from build123d import *

# Parameters (mm, degrees)
F0_R            = 31.75
F1_DEPTH        = 6.35
F2_R            = 4.7625
F3_DEPTH        = 6.351
F3_COPIES_COUNT = 6
F4_R            = 3.175
F5_R            = 3.175
F6_DEPTH        = 6.3510001
F6_COPIES_COUNT = 6
F7_R            = 9.4615
F7_R_2          = 7.9375
F8_DEPTH        = 9.7028
F8_COPIES_COUNT = 6


# Not quite as in the source:
# - a pattern or mirror of a feature is missing from the dataset's text; its kind, count and spacing are read off the source's solid


with BuildPart() as f1:
    # F0 (on Front) → F1 (new body)
    with BuildSketch(Plane.XZ):
        Circle(F0_R)
    extrude(amount=F1_DEPTH)

    # F2 (on face) → F3 (cut, through all)
    with BuildSketch(Plane.XZ.offset(6.35)):
        with Locations((-15.875, 27.4963065702)):
            Circle(F2_R)
    f3 = extrude(amount=-F3_DEPTH, mode=Mode.SUBTRACT)

    # F3_copies: F3 ×6 about axis
    f3_copies_axis = Axis((0, 0, 0), (0, 1, 0))
    for i in range(1, F3_COPIES_COUNT):
        add(f3.rotate(f3_copies_axis, i * 360 / F3_COPIES_COUNT), mode=Mode.SUBTRACT)

    # F4
    f4_edges = [f1.edges().sort_by_distance(p)[0] for p in [
        (-19.809236, -3.175, 24.81243),
        (-11.583577, -3.175, 29.561516),
        (-31.392813, -3.175, 4.749087),
        (11.583577, -3.175, 29.561516),
        (19.809236, -3.175, 24.81243),
        (31.392813, -3.175, 4.749087),
        (31.392813, -3.175, -4.749087),
        (19.809236, -3.175, -24.81243),
        (11.583577, -3.175, -29.561516),
        (-11.583577, -3.175, -29.561516),
        (-19.809236, -3.175, -24.81243),
        (-31.392813, -3.175, -4.749087),
    ]]
    fillet(f4_edges, radius=F4_R)

    # F5 (on face) → F6 (cut, through all)
    with BuildSketch(Plane.XZ.offset(6.35)):
        with Locations((0, 20.6375)):
            Circle(F5_R)
    f6 = extrude(amount=-F6_DEPTH, mode=Mode.SUBTRACT)

    # F6_copies: F6 ×6 about axis
    f6_copies_axis = Axis((0, 0, 0), (0, 1, 0))
    for i in range(1, F6_COPIES_COUNT):
        add(f6.rotate(f6_copies_axis, i * 360 / F6_COPIES_COUNT), mode=Mode.SUBTRACT)

    # F7 (on face) → F8 (join)
    with BuildSketch(Plane.XZ.offset(6.35)):
        with Locations((0, 20.6375)):
            Circle(F7_R)
        with Locations((0, 20.6375)):
            Circle(F7_R_2, mode=Mode.SUBTRACT)
    f8 = extrude(amount=F8_DEPTH)

    # F8_copies: F8 ×6 about axis
    f8_copies_axis = Axis((0, 0, 0), (0, 1, 0))
    for i in range(1, F8_COPIES_COUNT):
        add(f8.rotate(f8_copies_axis, i * 360 / F8_COPIES_COUNT))


solid = f1.part
CAD build for the part. Positions are in the model's coordinates, mm. A direction names the side the tool comes from. Give positions to 0.01 mm unless a question says otherwise; leave off trailing zeros. Write each loop counter-clockwise with the first axis right and the second up, starting at its lowest first coordinate (ties: lowest second). Pieces come first, ordered by that corner, then holes. Notation, with made-up numbers: (-10, 75.25) -> (26, 75.25) arc R29 ccw to (26, 106.25) -> close; hole circle Ø11 at (-30, -14.5). An arc over 180 degrees is marked (long way). Return JSON: item names as keys, results as strings.
Item 1: Band-saw the part on C-C (z = -26). List the corners of the cut face in (x, y).
Answer below:
{"outline": "(-11.35, -6.35) -> (-7.8, -6.35) -> (-7.8, -16.05) -> (-5.85, -16.05) -> (-5.85, -6.35) -> (5.85, -6.35) -> (5.85, -16.05) -> (7.8, -16.05) -> (7.8, -6.35) -> (11.35, -6.35) -> (11.35, 0) -> (-11.35, 0) -> close"}
Item 2: Band-saw the part on A-A (y = -9.5). Give the number of separate pieces and of enclosed holes in the cut face, then the cut area to 3 significant figures.
Answer below:
{"separate pieces": "6", "enclosed holes": "6", "area": "500 mm2"}
Item 3: Two-plate mould, pull along Z, no slides. Class faces 3 (the cylindrical face through (-14.94, -3.219, -11.535)), 4 (the cylindrical face through (-0.13, -3.13, -31.75)), 5 (the flat face through (5, -16.053, -27)): +Z half, -Z half, draft (parallel to the pull), parting line (faces both ways), or undercut.
Answer below:
{"face 3": "undercut", "face 4": "-Z half", "face 5": "draft"}
Item 4: Drill centre lines: probe 1 along Z at (x, y) = (0, -1.5); probe 2 along Z at (x, y) = (-13, -10); probe 3 along Z at (x, y) = (3, -10.5). Where is each one in solid material? Low to high.
Answer below:
{"probe 1": "z = -31.75 to -23.81, -17.46 to 17.46, 23.81 to 31.75", "probe 2": "z = -18.43 to -16.58, -4.05 to -2.21, 2.21 to 4.05, 16.58 to 18.43", "probe 3": "z = -29.61 to -27.99, -13.29 to -11.66, 11.66 to 13.29, 27.99 to 29.61"}
Item 5: Drop flat-ended pins along their axis: pin 1 (3 mm diameter, centred on y = -3, z = -22, fed in from +X); pin 2 (8.5 mm diameter, centred on x = 0, z = -20.64, fed in from -Y); pin 3 (2 mm diameter, centred on x = 2.5, y = -9, fed in from +Z); pin 4 (4 mm diameter, centred on x = 17.87, z = -10.32, fed in from +Y). Give the stop position or say it passes through.
Answer below:
{"pin 1": "stops at x = 24.24", "pin 2": "stops at y = -6.35", "pin 3": "stops at z = 29.98", "pin 4": "passes through"}
Item 6: Tool access for faces 1 (the cylindrical face through (-1.72, -11.13, 12.89)), 2 (the cylindrical face through (13.43, -3.22, 23.41)): list every direction of +Z, -Z, +X, -X, +Y, -Y with a clear straight run to the whole face (end or side of a thin tool).
Answer below:
{"face 1": "-Y", "face 2": "+Z, +Y, -Y"}
